The model under review builds one solid part; all positions refer to its coordinate system, in mm. A direction names the side the tool comes from. Give positions to 0.01 mm unless a question says otherwise; leave off trailing zeros. Loops run counter-clockwise (first coordinate to the right, second up) from the corner with the lowest first, then second, coordinate; pieces in that order, holes last. Notation, with made-up numbers: (87.5, -24.5) - (124.5, -24.5) arc R32 ccw to (124.5, 6.5) - close; hole circle Ø4 at (-3, -33.75). An arc over 180 degrees is marked (long way). Return JSON: item names as keys, results as strings. Group by question number.
from build123d import *

# Parameters (mm, degrees)
F1_DEPTH = 21.43125
F2_R     = 9.525
F3_DEPTH = 50.8
F5_DEPTH = 42.8635


with BuildPart() as f1:
    # F0 (on Right) → F1 (new body, symmetric)
    with BuildSketch(Plane.YZ):
        Polygon((-152.4, 69.85), (-152.4, 0), (152.4, 0), (152.4, 19.05), align=None)
    extrude(amount=F1_DEPTH, both=True)

    # F2 (on face) → F3 (cut)
    with BuildSketch(Plane.XZ.offset(152.4)):
        with Locations((0, 34.925)):
            Circle(F2_R)
    extrude(amount=-F3_DEPTH, mode=Mode.SUBTRACT)

    # F4 (on face) → F5 (intersect, through all)
    with BuildSketch(Plane.YZ.offset(21.43125)):
        Polygon((-16.6460395549, 45.5284491181), (-48.7253032625, 45.5284491181), (-48.6101253426, 28.6297574639), (-48.5881119967, 25.4), (-48.7253032625, 25.4), (-95.2500006139, 25.4), (-95.2500006139, 50.7999987721), (-152.4, 50.7999987721), (-152.4, 9.525), (-127, 9.525), (18.3262217238, 9.525), (37.3762217238, 9.525), (37.3762217238, 28.6172106862), (0, 28.6172106862), align=None)
        with BuildLine():
            ThreePointArc((-125.4125, 19.05), (-125.8774679849, 17.9274679849), (-127, 17.4625))
            ThreePointArc((-127, 17.4625), (-128.1225320151, 20.1725320151), (-125.4125, 19.05))
        make_face(mode=Mode.SUBTRACT)
        with BuildLine():
            ThreePointArc((19.9137217238, 19.05), (19.448753739, 17.9274679849), (18.3262217238, 17.4625))
            ThreePointArc((18.3262217238, 17.4625), (17.2036897087, 20.1725320151), (19.9137217238, 19.05))
        make_face(mode=Mode.SUBTRACT)
    extrude(amount=-F5_DEPTH, mode=Mode.INTERSECT)


solid = f1.part
Item 1: Take a section at D-D (y = -117). State the section outline as (x, z) points (3 decimals), then the cut area to 3 significant figures.
Item 2: For L1, parallel to Y at x = -6, z = 19.05; L2, parallel to Z at x = 0, y = -111 (3 decimals); L3, parallel to Y at x = 15.5, z = 18.5, list the stretches that pass through material, from the lowest coordinate up. Write a range as from..to.
Item 3: Take a section at B-B (y = -27.5). State the section outline as (x, z) points (3 decimals).
Item 4: Tool access review of faces 5 (the face through (0, -59, 9.525)), 6 (the face through (0, -95.25, 38)), 7 (the face through (0, 19, 28.617)): name each direction out of +Z, -Z, +X, -X, +Y, -Y from which nothing blocks a thin tool from reaching the whole face with its end or side.
Item 5: For P1, Ø1, axis at x = 3.5, y = -16.5, coming from the +Z side; P2, Ø7.5, axis at x = 7, z = 33.5, coming from the +Y side (3 decimals); P3, Ø8, axis at x = -12, z = 40.5, coming from the +Y side; P4, Ø1.9, axis at y = 18.33, z = 19.05, coming from the +X side, all flat-tipped, find the tip position at first contact; note any pin that passes through.
Item 6: Take a section at A-A (x = 0). State how many separate pieces and enclosed holes the cut face has, then the cut area to 3 significant figures.
Item 7: Mouldability with a two-part tool opening along X and no side actions: class faces 1 (the face through (0.3, -8.206, 36.954)), 2 (the face through (-1.24, -127.36, 44.37)), 3 (the face through (0, -101.6, 35)), 4 (the face through (21.431, -80, 21)) as +X half, -X half, draft (parallel to the pull), parting line (faces both ways), or undercut.
Check sheet entries:
{
 "1": {"outline": "(-21.431, 9.525) - (21.431, 9.525) - (21.431, 50.8) - (-21.431, 50.8) - close; hole circle Ø19.05 at (0, 34.925)", "area": "1,480 mm^2"},
 "2": {"L1": "y = -152.4..-128.59, -125.41..16.74, 19.91..37.38", "L2": "z = 9.525..25.4, 44.45..50.8", "L3": "y = -152.4..-128.49, -125.51..16.84, 19.82..37.38"},
 "3": {"outline": "(-21.431, 9.525) - (21.431, 9.525) - (21.431, 45.528) - (-21.431, 45.528) - close"},
 "4": {"face 5": "-Z, +X, -X, +Y, -Y", "face 6": "+Z, +X, -X", "face 7": "+Z, +X, -X, +Y"},
 "5": {"P1": "stops at z = 45.53", "P2": "stops at y = -1.115", "P3": "stops at y = -7.76", "P4": "passes through"},
 "6": {"separate pieces": "1", "enclosed holes": "2", "area": "4,440 mm^2"},
 "7": {"face 1": "draft", "face 2": "undercut", "face 3": "undercut", "face 4": "+X half"}
}
